CAD build for the part. Positions are in the model's coordinates, mm. A direction names the side the tool comes from. Give positions to 0.01 mm unless a question says otherwise; leave off trailing zeros. Answer as CSV lines item,"result".
from build123d import *

# Parameters (mm, degrees)
SKETCH1_W                      = 600
SKETCH1_H                      = 245
BOSS_EXTRUDE1_DEPTH            = 19.05
CBORE_FOR_M5_SHCS1_D           = 5
CBORE_FOR_M5_SHCS1_DEPTH       = 28.497848452
CBORE_FOR_M5_SHCS1_CBORE_D     = 10
CBORE_FOR_M5_SHCS1_CBORE_DEPTH = 5
CBORE_FOR_M5_SHCS1_TIP         = 1.502151548


with BuildPart() as part:
    # Sketch1 → Boss-Extrude1 (new body)
    with BuildSketch(Plane.XY):
        with Locations((0, 127.5)):
            Rectangle(SKETCH1_W, SKETCH1_H)
    extrude(amount=BOSS_EXTRUDE1_DEPTH)

    # CBORE for M5 SHCS1
    with Locations(Plane.XY.offset(19.05)):
        with Locations((-270, 215), (-210, 215), (-150, 215), (-90, 215), (-30, 215), (30, 215), (90, 215), (150, 215), (210, 215), (270, 215), (270, 155), (270, 95), (90, 155), (90, 95), (-30, 155), (-30, 95), (-150, 155), (-270, 155), (-270, 95), (-150, 95), (-270, 35), (-210, 35), (-150, 35), (-90, 35), (-30, 35), (30, 35), (90, 35), (150, 35), (210, 35), (270, 35)):
            CounterBoreHole(CBORE_FOR_M5_SHCS1_D / 2, CBORE_FOR_M5_SHCS1_CBORE_D / 2, CBORE_FOR_M5_SHCS1_CBORE_DEPTH, depth=CBORE_FOR_M5_SHCS1_DEPTH)
            with Locations((0, 0, -(CBORE_FOR_M5_SHCS1_DEPTH + CBORE_FOR_M5_SHCS1_TIP / 2))):  # 118° drill point
                Cone(0, CBORE_FOR_M5_SHCS1_D / 2, CBORE_FOR_M5_SHCS1_TIP, mode=Mode.SUBTRACT)


solid = part.part
1) Which spindle directions (+Z, -Z, +X, -X, +Y, -Y) get a long thin tool onto all of the face, cutting with end or side? Do faces 1 (the face through (-4, 129, 19.05)), 2 (the face through (-148, 33, 14.05)). Say none if no direction does.
Answer below:
face 1,"+Z, +X, -X, +Y, -Y"
face 2,"+Z"
2) Flat gauge pins, fed straight in: pin 1 (6 mm diameter, centred on x = -30, y = 95, fed in from -Z); pin 2 (6 mm diameter, centred on x = -150, y = 35, fed in from +Z). Where does each tip first touch, or does it go through?
Answer below:
pin 1,"stops at z = 0"
pin 2,"stops at z = 14.05"
3) Drill centre lines: line 1 (Y direction, x = -270.5, z = 14.25); line 2 (Y direction, x = 270, z = 4.5); line 3 (X direction, y = 155, z = 5.25). Where is each one in solid material? Low to high. Write a range as from..to.
Answer below:
line 1,"y = 5..30.03, 39.97..90.03, 99.97..150.03, 159.97..210.03, 219.97..250"
line 2,"y = 5..32.5, 37.5..92.5, 97.5..152.5, 157.5..212.5, 217.5..250"
line 3,"x = -300..-272.5, -267.5..-152.5, -147.5..-32.5, -27.5..87.5, 92.5..267.5, 272.5..300"
4) Mould opens along Y. For faces 3 (the face through (-4, 129, 0)), 4 (the face through (214.77, 36.5, 16.58)), 5 (the face through (-4, 250, 9)), 6 (the face through (-30.651, 219.957, 16.585)) say: +Y half, -Y half, draft (parallel to the pull), parting line (faces both ways), or undercut.
Answer below:
face 3,"draft"
face 4,"undercut"
face 5,"+Y half"
face 6,"undercut"
